Autodesk Fusion 360 part; units mm, degrees
ref_plane "WorkPlane1" through (0, 12, 0) normal (0, 1, 0) x (0, 0, 1)
sketch "Sketch1" plane through (0, 0, 0) normal (0, 1, 0) x (1, 0, 0)
  circle A0 centre (0, 0) radius 1.65
  circle A1 centre (0, 0) radius 4
  circle A2 centre (0, 77) radius 1.65
  circle A3 centre (0, 77) radius 4
  circle A4 centre (62, 0) radius 1.65
  circle A5 centre (62, 0) radius 4
  circle A6 centre (62, 77) radius 4
  circle A7 centre (62, 77) radius 1.65
  line L0 (-7, 84) -> (69, 84)
  line L1 (69, 84) -> (69, -7)
  line L2 (69, -7) -> (-7, -7)
  line L3 (-7, -7) -> (-7, 84)
  line L4 (4, 73) -> (58, 73)
  line L5 (58, 73) -> (58, 4)
  line L6 (58, 4) -> (4, 4)
  line L7 (4, 4) -> (4, 73)
  line L8 (-7, -52) -> (4, -52)
  line L9 (4, -52) -> (4, -7)
  line L10 (4, -7) -> (-7, -7)
  line L11 (-7, -7) -> (-7, -52)
  line L12 (69, -7) -> (58, -7)
  line L13 (58, -7) -> (58, -52)
  line L14 (58, -52) -> (69, -52)
  line L15 (69, -52) -> (69, -7)
  line L16 (-7, -20) -> (69, -20)
  line L17 (69, -20) -> (69, -52)
  line L18 (69, -52) -> (-7, -52)
  line L19 (-7, -52) -> (-7, -20)
  dimension "d1" = 3.3
  dimension "d2" = 8
  dimension "d3" = 3.3
  dimension "d4" = 8
  dimension "d5" = 77
  dimension "d6" = 3.3
  dimension "d7" = 8
  dimension "d8" = 62
  dimension "d9" = 3.3
  dimension "d10" = 8
  dimension "d11" = 77
  dimension "d12" = 7
  dimension "d13" = 7
  dimension "d14" = 7
  dimension "d15" = 7
  dimension "d16" = 4
  dimension "d17" = 4
  dimension "d18" = 4
  dimension "d19" = 4
  dimension "d52" = 45
  dimension "d53" = 11
  dimension "d54" = 45
  dimension "d55" = 11
  dimension "d65" = 20
extrude "Extrude1" add sketch "Sketch1" along normal blind 3 contours L0 L1 L2 L3 L10 L12 | L2 L9 L10 L11 L16 | L2 L12 L13 L15 L16 | L8 L9 L11 L16 L18 L19 | L13 L14 L15 L16 L17 L18
extrude "Extrude2" add sketch "Sketch1" along normal blind 2 contours A1 | A3 | A5 | A6
sketch "Sketch3" plane through (0, 0, 0) normal (1, 0, 0) x (0, 0, -1)
  circle A0 centre (32, 7) radius 1.65
  circle A1 centre (32, 7) radius 3.75
  line L0 (84, 0) -> (-52, 0)
  line L1 (77, 0) -> (32, 0)
  line L2 (39, 12) -> (25, 12)
  line L3 (25, 12) -> (25, 3)
  line L4 (25, 3) -> (39, 3)
  line L5 (39, 3) -> (39, 12)
  line L6 (4, 3) -> (73, 3)
  circle A2 centre (-45, 7) radius 1.65
  circle A3 centre (-45, 7) radius 3.75
  line L7 (32, 0) -> (-45, 0)
  line L8 (-38, 12) -> (-52, 12)
  line L9 (-52, 12) -> (-52, 0)
  line L10 (-52, 0) -> (-38, 0)
  line L11 (-38, 0) -> (-38, 12)
  line L12 (-7, 0) -> (-52, 0)
  point P0 (77, 0)
  dimension "d24" = 3.3
  dimension "d25" = 7.5
  dimension "d27" = 45
  dimension "d28" = 7
  dimension "d29" = 5
  dimension "d30" = 7
  dimension "d31" = 7
  dimension "d32" = 3.3
  dimension "d33" = 7.5
  dimension "d34" = 77
  dimension "d35" = 7
  dimension "d36" = 5
  dimension "d37" = 7
  dimension "d38" = 7
extrude "Extrude3" add sketch "Sketch3" along normal blind 3 from surface at -7 contours L0 L7 L8 L9 L10 L11 L12 | L2 L3 L4 L5 L6
extrude "Extrude5" add sketch "Sketch3" along normal blind 2 from surface at -6 contours A1 | A3
extrude "Extrude6" add sketch "Sketch3" along normal blind 3 from surface at 66 contours L0 L7 L8 L9 L10 L11 L12 | L2 L3 L4 L5 L6
extrude "Extrude7" add sketch "Sketch3" along normal blind 2 from surface at 66 contours A1 | A3
fillet "Fillet1" radius 4.5 4 edges at (-7, 1.5, -84) (69, 1.5, -84) (4, 1.5, 52) (58, 1.5, 52)
fillet "Fillet2" radius 4.5 6 edges at (4, 1.5, -73) (4, 1.5, -4) (58, 1.5, -4) (58, 1.5, -73) (4, 1.5, 7) (58, 1.5, 7)
extrude "Extrude8" cut sketch "Sketch1" along normal blind 1 contours L8 L9 L11 L16 L18 L19 | L13 L14 L15 L16 L17 L18 | L9 L13 L16 L18
fillet "Fillet3" radius 3.5 8 edges at (67.5, 12, -25) (-5.5, 12, -25) (-5.5, 12, 52) (-5.5, 12, 38) (67.5, 12, 52) (67.5, 12, 38) (67.5, 12, -39) (-5.5, 12, -39)
Design review of the part built by this model. Coordinates are the model's own, in mm. A direction names the side the tool comes from. Give positions to 0.01 mm unless a question says otherwise; leave off trailing zeros. Loops run counter-clockwise (first coordinate to the right, second up) from the corner with the lowest first, then second, coordinate; pieces in that order, holes last. Notation, with made-up numbers: M 40.25,20 L 71.25,20 A30 cw 71.25,56 Z; hole C 19.25,14 d9. An arc over 180 degrees is marked long. Return JSON: item names as keys, results as strings. Group by question number.
Item 1: For probe 1 along X at (y, z) = (1.25, 0); probe 2 along X at (y, z) = (2.2, -77); probe 3 along Z at (x, y) = (0, 2.5), list the stretches that pass through material, from the lowest coordinate up.
Item 2: We need section C-C (z = -19.5). Give the boundary of the cut face in (x, y), and give its area (3 significant figures).
Item 3: Insertion check: pin 1 Ø4 at (y, z) = (6.5, 44) entering from +X; pin 2 Ø6 at (x, z) = (52.5, -24.5) entering from +Y; pin 3 Ø2.5 at (x, z) = (0.5, -77.5) entering from +Y; pin 4 Ø3.5 at (x, z) = (66, 29) entering from -Y. Each pin has a flat end and moves straight along its axis. Give the tip position at first contact, or say it passes through.
Item 4: We need section D-D (z = 0). Give the boundary of the cut face in (x, y), and give its area (3 significant figures).
Item 5: We need section B-B (x = 48). Give the boundary of the cut face in (y, z).
Item 6: Mouldability with a two-part tool opening along Z and no side actions: class faces 6 (the flat face through (31, 1, -73)), 7 (the cylindrical face through (60.35, 0.99, -76.93)), 8 (the flat face through (-6, 12, 45)), 9 (the flat face through (-5, 4, 52)) as released by +Z, released by -Z, zero draft, split by the parting line, or undercut.
Item 7: Tool access review of faces 1 (the flat face through (-4, 8, 47)), 2 (the flat face through (31, 1, 7)), 3 (the flat face through (-6, 6, 38)), 4 (the flat face through (68, 6, 43)), 5 (the cylindrical face through (-0.867, 2.493, -80.905)): name each direction out of +Z, -Z, +X, -X, +Y, -Y from which nothing blocks a thin tool from reaching the whole face with its end or side.
Item 8: We need section A-A (z = 45). Give the boundary of the cut face in (x, y), and give its area (3 significant figures).
Output:
{
 "1": {"probe 1": "x = -7 to -1.65, 1.65 to 60.35, 63.65 to 69", "probe 2": "x = -7 to -4, 4 to 58, 66 to 69", "probe 3": "z = -84 to -81, -73 to -4, 4 to 51.97"},
 "2": {"outline": "M -7,0 L 4,0 L 4,3 L -7,3 Z; M 58,0 L 69,0 L 69,3 L 58,3 Z", "area": "66.0 mm^2"},
 "3": {"pin 1": "stops at x = 68", "pin 2": "passes through", "pin 3": "stops at y = 2", "pin 4": "stops at y = 1"},
 "4": {"outline": "M -7,0 L -1.65,0 L -1.65,2 L -4,2 L -4,3 L -7,3 Z; M 1.65,0 L 60.35,0 L 60.35,2 L 58,2 L 58,3 L 4,3 L 4,2 L 1.65,2 Z; M 63.65,0 L 69,0 L 69,3 L 66,3 L 66,2 L 63.65,2 Z", "area": "199 mm^2"},
 "5": {"outline": "M 0,-84 L 3,-84 L 3,-73 L 0,-73 Z; M 0,-4 L 3,-4 L 3,7 L 0,7 Z"},
 "6": {"face 6": "undercut", "face 7": "undercut", "face 8": "zero draft", "face 9": "released by +Z"},
 "7": {"face 1": "+Z, -Z, +Y", "face 2": "+Z, +Y, -Y", "face 3": "+X, -X, +Y", "face 4": "+X", "face 5": "+Y"},
 "8": {"outline": "M -7,1 L 4,1 L 4,3 L -4,3 L -4,5.35 L -6,5.35 L -6,3.25 L -7,3.25 Z; M -7,10.75 L -6,10.75 L -6,8.65 L -4,8.65 L -4,12 L -7,12 Z; M 58,1 L 69,1 L 69,3.25 L 68,3.25 L 68,5.35 L 66,5.35 L 66,3 L 58,3 Z; M 66,8.65 L 68,8.65 L 68,10.75 L 69,10.75 L 69,12 L 66,12 Z", "area": "69.8 mm^2"}
}
